Print and shaded views of the part. All mm, measured from the part's lowest x, y and z. Give positions to 0.01 mm unless a question says otherwise; leave off trailing zeros. Order: outer loops, then holes, each group sorted by start corner. A loop starts at its lowest first (then second) coordinate and runs counter-clockwise, first axis right, second up. Notation, with made-up numbers: (-19, 84) -> (-7, 84) arc R13 ccw to (-7, 96) -> close; hole circle Ø8 at (50.25, 47). An arc over 180 degrees is marked (long way). One line per question, with ' | ' between items. Start each with the question number.
(1) Cut at B-B (y = 15). Give the cut face in (x, z).
(2) Drill centre lines: L1, parallel to X at y = 15, z = 1.3; L2, parallel to Y at x = 15, z = 1; L3, parallel to X at y = 18, z = 2.05. Where is each one in solid material? Low to high. Write a range as from..to.
(3) Cut at A-A (x = 15). Give the cut face in (y, z), then the cut area to 3 significant figures.
(4) Cut at C-C (z = 0.45). Give the cut face in (x, y), then the cut area to 3 significant figures.
(5) Pull direction X, two halves, no side cores. Call the marked faces 1 and 2: +X half, -X half, draft (parallel to the pull), parting line (faces both ways), or undercut.
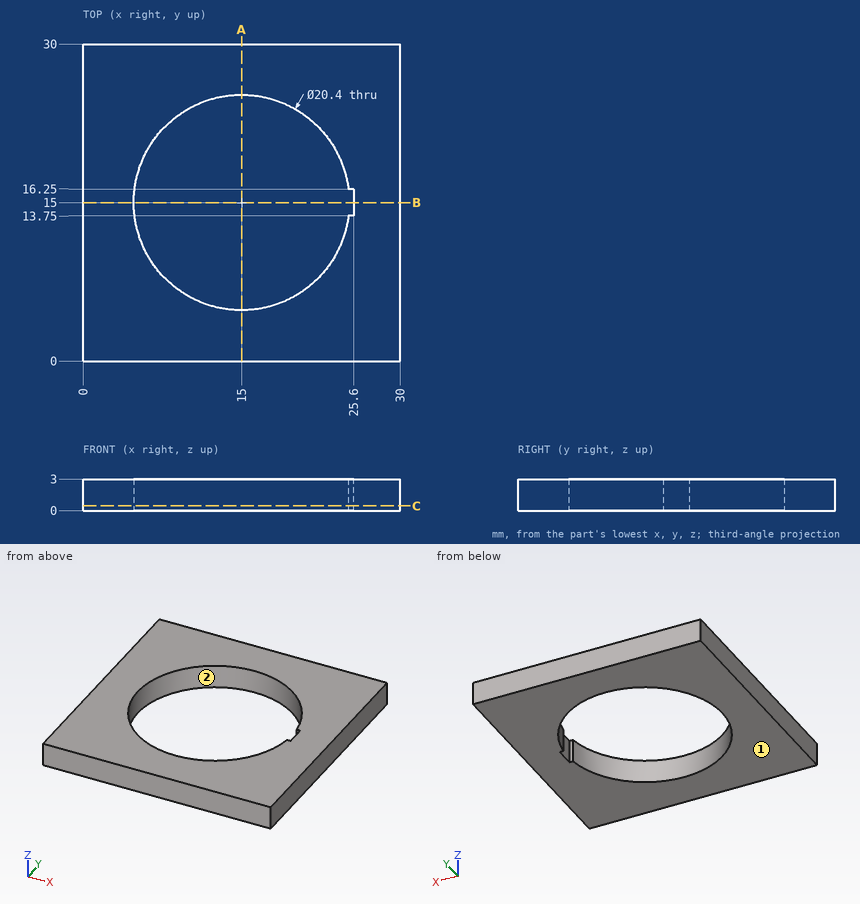
Result set:
1) outline: (0, 0) -> (4.8, 0) -> (4.8, 3) -> (0, 3) -> close; (25.6, 0) -> (30, 0) -> (30, 3) -> (25.6, 3) -> close
2) L1: x = 0..4.8, 25.6..30 | L2: y = 0..4.8, 25.2..30 | L3: x = 0..5.25, 24.75..30
3) outline: (0, 0) -> (4.8, 0) -> (4.8, 3) -> (0, 3) -> close; (25.2, 0) -> (30, 0) -> (30, 3) -> (25.2, 3) -> close | area: 28.8 mm2
4) outline: (0, 0) -> (30, 0) -> (30, 30) -> (0, 30) -> close; hole (25.12, 13.75) -> (25.6, 13.75) -> (25.6, 16.25) -> (25.12, 16.25) arc R10.2 ccw (long way) to start | area: 572 mm2
5) face 1: draft | face 2: undercut
